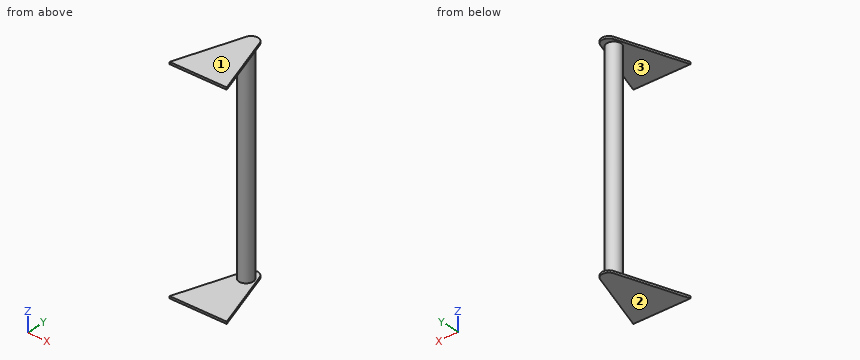
Autodesk Inventor part; units mm, degrees
ref_plane "YZ Plane" through (0, 0, 0) normal (1, 0, 0) x (0, 1, 0)
ref_plane "XZ Plane" through (0, 0, 0) normal (0, 1, 0) x (-1, 0, 0)
ref_plane "XY Plane" through (0, 0, 0) normal (0, 0, 1) x (1, 0, 0)
sketch "Sketch1" plane through (0, 0, 0) normal (0, 0, 1) x (1, 0, 0)
  point P0 (0, 0)
sketch "Sketch2" plane through (0, 0, 0) normal (0, 0, 1) x (1, 0, 0)
  line L0 (0, 0) -> (80, 0)
  line L1 (80, 0) -> (40, 120)
  line L2 (40, 120) -> (0, 0)
  dimension "d0" = 80
  dimension "d1" = 120
  dimension "d2" = 40
extrude "Extrusion1" add sketch "Sketch2" against normal blind 3
sketch "Sketch3" plane through (0, 0, -3) normal (0, 0, -1) x (-1, 0, 0)
  circle A0 centre (-40, 80) radius 10
  line L0 (-80, 0) -> (0, 0)
  point P0 (-40, 120)
  point P1 (-40, 0)
  dimension "d5" = 20
  dimension "d6" = 0
  dimension "d7" = 80
fillet "Fillet1" radius 10 1 edges at (40, 120, -1.5)
extrude "Extrusion2" add sketch "Sketch3" along normal blind 147
mirror "Mirror1" about plane through (40, 80, -150) normal (0, 0, -1) of "Extrusion2", "Extrusion1"
fillet "Fillet2" radius 10 1 edges at (40, 120, -298.5)
properties part number "stand"
Verification items for the finished model (mm, model axes). Face numbers are marked on the shaded views. Give positions to 0.01 mm unless a question says otherwise; leave off trailing zeros. Loops run counter-clockwise (first coordinate to the right, second up) from the corner with the lowest first, then second, coordinate; pieces in that order, holes last. Notation, with made-up numbers: (43.5, 33) - (49.5, 33) arc R12 cw to (49.5, 53) - close; hole circle Ø5 at (16.5, -4). An arc over 180 degrees is marked (long way). Write item = value, one per line. Start each with the question number.
Q1. Cross-section at A-A, the plane x = 26.5. Enter the section's corners in (y, z), and give its area (3 significant figures).
Q2. Thickness scan on line 1 (Z direction, x = 37, y = 70); line 2 (Y direction, x = 40, z = -124.5); line 3 (X direction, y = 83, z = -152). Record the ranges inside material, lowest first.
Q3. Mould release check, pull along Z, two halves, no side actions. Record for the marked faces 1, 2 and 3: released by +Z, released by -Z, zero draft, split by the parting line, or undercut.
Q4. Cross-section at D-D, the plane x = 40. Enter the section's corners in (y, z), and give its area (3 significant figures).
Q5. Cross-section at B-B, the plane y = 28.5. Enter the section's corners in (x, z), and give its area (3 significant figures).
Q6. Depth check by flat-ended pin: P1, Ø4, axis at y = 70.5, z = -192, coming from the +X side; P2, Ø5, axis at y = 70.5, z = -106, coming from the -X side; P3, Ø4, axis at x = 48.5, y = 52.5, coming from the +Z side. Enter the tip coordinate at first touch or a pass-through.
Q7. Cross-section at C-C, the plane z = -262.5. Enter the section's corners in (x, y).
Answer key:
q1.outline = (0, -300) - (79.5, -300) - (79.5, -297) - (0, -297) - close; (0, -3) - (79.5, -3) - (79.5, 0) - (0, 0) - close
q1.area = 477 mm^2
q2.line_1 = -300 to -297, -3 to 0
q2.line_2 = 70 to 90
q2.line_3 = 30.46 to 49.54
q3.face_1 = released by +Z
q3.face_2 = released by -Z
q3.face_3 = undercut
q4.outline = (0, -300) - (98.38, -300) - (98.38, -297) - (90, -297) - (90, -3) - (98.38, -3) - (98.38, 0) - (0, 0) - (0, -3) - (70, -3) - (70, -297) - (0, -297) - close
q4.area = 6,470 mm^2
q5.outline = (9.5, -300) - (70.5, -300) - (70.5, -297) - (9.5, -297) - close; (9.5, -3) - (70.5, -3) - (70.5, 0) - (9.5, 0) - close
q5.area = 366 mm^2
q6.P1 = 46.61
q6.P2 = 32.86
q6.P3 = 0
q7.outline = circle Ø20 at (40, 80)
